Read the model definition and answer for the solid it produces. Units are mm, in the model's axes. Round coordinates to 2 decimals unless told otherwise and drop trailing zeros. Write each loop counter-clockwise with the first axis right and the second up, starting at its lowest first coordinate (ties: lowest second). Pieces come first, ordered by that corner, then holes. Notation, with made-up numbers: (61, 17.5) -> (101, 17.5) arc R30 cw to (101, 51.5) -> close; hole circle Ø2 at (-8, -4.5). An arc over 180 degrees is marked (long way). Return JSON: item names as keys, results as strings. Group by question number.
(1) A cutting plane is placed at A-A on y = -65.65. Give the vertices of the cut face in (x, z).
(2) Straight lines are drawn through the part: line 1 (Y direction, x = -29, z = 2.6); line 2 (X direction, y = 42, z = 0.6); line 3 (X direction, y = 22, z = 2.25). For each, find the intervals that lie inside material, in ascending order.
(3) A cutting plane is placed at B-B on x = 4. Give the vertices of the cut face in (y, z).
(4) A cutting plane is placed at C-C on x = -16.5. Give the vertices of the cut face in (y, z).
(5) A cutting plane is placed at D-D on z = 0.7. Give the vertices of the cut face in (x, y) (3 decimals), then the cut area to 3 significant figures.
(6) Given pin 1 (1.9 mm diameter, centred on x = -53.71, y = -73.35, fed in from -Z); pin 2 (5 mm diameter, centred on x = -53.71, y = 73.35, fed in from +Z), each flat-ended and moving along its own axis, determine where each tip first touches the part or whether it passes through.
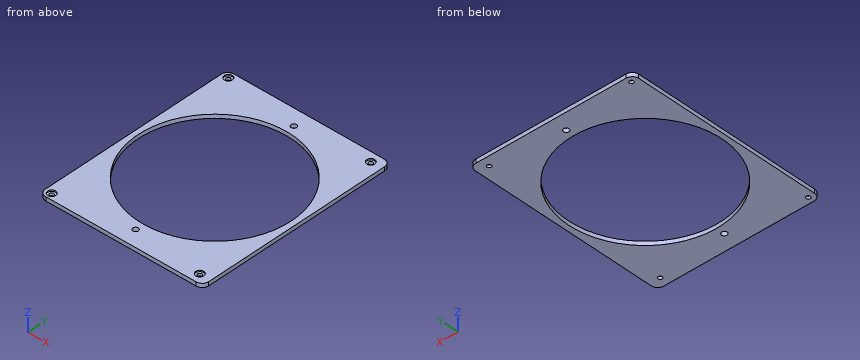
```python
from build123d import *

# Parameters (mm, degrees)
SKETCH_1_R          = 59.1
SKETCH_1_R_2        = 1.6
EXTRUDE_1_DEPTH     = 3
SKETCH_2_R          = 2.1
CUT_EXTRUDE_1_DEPTH = 104.064494371
SKETCH_3_R          = 3.1
CUT_EXTRUDE_2_DEPTH = 1


with BuildPart() as part:
    # 草图1 → 凸台-拉伸1 (new body)
    with BuildSketch(Plane.XY):
        with BuildLine():
            Line((62.3, -78), (-53.9, -78))
            ThreePointArc((-53.9, -78), (-57.435533906, -76.535533906), (-58.9, -73))
            Line((-58.9, -73), (-58.9, 73))
            ThreePointArc((-58.9, 73), (-57.435533906, 76.535533906), (-53.9, 78))
            Line((-53.9, 78), (62.3, 78))
            ThreePointArc((62.3, 78), (65.835533906, 76.535533906), (67.3, 73))
            Line((67.3, 73), (67.3, -73))
            ThreePointArc((67.3, -73), (65.835533906, -76.535533906), (62.3, -78))
        make_face()
        with Locations((4, 0)):
            Circle(SKETCH_1_R, mode=Mode.SUBTRACT)
        with Locations((58.493442579, 70.964337058)):
            Circle(SKETCH_1_R_2, mode=Mode.SUBTRACT)
        with Locations((-53.705008218, 73.348219362)):
            Circle(SKETCH_1_R_2, mode=Mode.SUBTRACT)
        with Locations(Location((58.493442579, -70.964337058, 0), (0, 0, 180))):
            Circle(SKETCH_1_R_2, mode=Mode.SUBTRACT)
        with Locations(Location((-53.705008218, -73.348219362, 0), (0, 0, 180))):
            Circle(SKETCH_1_R_2, mode=Mode.SUBTRACT)
    extrude(amount=EXTRUDE_1_DEPTH)

    # 草图2 → 切除-拉伸1 (cut, through all)
    with BuildSketch(Plane.XY.offset(3)):
        with Locations((4, -65.65)):
            Circle(SKETCH_2_R)
        with Locations((4, 65.65)):
            Circle(SKETCH_2_R)
    extrude(amount=-CUT_EXTRUDE_1_DEPTH, mode=Mode.SUBTRACT)

    # 草图3 → 切除-拉伸2 (cut)
    with BuildSketch(Plane.XY.offset(3)):
        with Locations((58.493442579, -70.964337058)):
            Circle(SKETCH_3_R)
        with Locations((-53.705008218, -73.348219362)):
            Circle(SKETCH_3_R)
        with Locations(Location((-53.705008218, 73.348219362, 0), (0, 0, 180))):
            Circle(SKETCH_3_R)
        with Locations(Location((58.493442579, 70.964337058, 0), (0, 0, 180))):
            Circle(SKETCH_3_R)
    extrude(amount=-CUT_EXTRUDE_2_DEPTH, mode=Mode.SUBTRACT)


solid = part.part
```
Checks:
{
 "1": {"outline": "(-58.9, 0) -> (1.9, 0) -> (1.9, 3) -> (-58.9, 3) -> close; (6.1, 0) -> (67.3, 0) -> (67.3, 3) -> (6.1, 3) -> close"},
 "2": {"line 1": "y = -78 to -49.03, 49.03 to 78", "line 2": "x = -58.9 to -37.58, 45.58 to 67.3", "line 3": "x = -58.9 to -50.85, 58.85 to 67.3"},
 "3": {"outline": "(-78, 0) -> (-67.75, 0) -> (-67.75, 3) -> (-78, 3) -> close; (-63.55, 0) -> (-59.1, 0) -> (-59.1, 3) -> (-63.55, 3) -> close; (59.1, 0) -> (63.55, 0) -> (63.55, 3) -> (59.1, 3) -> close; (67.75, 0) -> (78, 0) -> (78, 3) -> (67.75, 3) -> close"},
 "4": {"outline": "(-78, 0) -> (-55.43, 0) -> (-55.43, 3) -> (-78, 3) -> close; (55.43, 0) -> (78, 0) -> (78, 3) -> (55.43, 3) -> close"},
 "5": {"outline": "(-58.9, -73) arc R5 ccw to (-53.9, -78) -> (62.3, -78) arc R5 ccw to (67.3, -73) -> (67.3, 73) arc R5 ccw to (62.3, 78) -> (-53.9, 78) arc R5 ccw to (-58.9, 73) -> close; hole circle Ø3.2 at (-53.705, -73.348); hole circle Ø3.2 at (-53.705, 73.348); hole circle Ø118.2 at (4, 0); hole circle Ø4.2 at (4, -65.65); hole circle Ø4.2 at (4, 65.65); hole circle Ø3.2 at (58.493, -70.964); hole circle Ø3.2 at (58.493, 70.964)", "area": "8,630 mm^2"},
 "6": {"pin 1": "passes through", "pin 2": "stops at z = 2"}
}
